Part model, mm, in its own coordinate system. A direction names the side the tool comes from. Give positions to 0.01 mm unless a question says otherwise; leave off trailing zeros. Order: outer loops, then holes, each group sorted by start corner. A loop starts at its lowest first (then second) coordinate and runs counter-clockwise, first axis right, second up. Notation, with made-up numbers: M 19,51 L 30,51 A25 cw 30,82 Z; hole C 54,85.5 d1. An arc over 180 degrees is marked long. Return JSON: item names as keys, results as strings.
from build123d import *

# Parameters (mm, degrees)
F0_R     = 50.9
F0_R_2   = 40.9
F1_DEPTH = 12.7
F2_R     = 5
F3_R     = 42.5
F4_DEPTH = 10
F5_R     = 42.5
F6_DEPTH = 10
F7_R     = 9.779
F8_DEPTH = 5.4


with BuildPart() as f1:
    # F0 (on Front) → F1 (new body, symmetric)
    with BuildSketch(Plane.XZ):
        Circle(F0_R)
        Circle(F0_R_2, mode=Mode.SUBTRACT)
        Circle(F0_R_2)
    extrude(amount=F1_DEPTH, both=True)

    # F2
    f2_edges = [f1.edges().sort_by_distance(p)[0] for p in [
        (-50.9, -12.7, 0),
        (-50.9, 12.7, 0),
    ]]
    fillet(f2_edges, radius=F2_R)

    # F3 (on face) → F4 (cut)
    with BuildSketch(Plane.XZ.offset(12.7)):
        Circle(F3_R)
    extrude(amount=-F4_DEPTH, mode=Mode.SUBTRACT)

    # F5 (on face) → F6 (cut)
    with BuildSketch(Plane(origin=(0, 12.7, 0), x_dir=(-1, 0, 0), z_dir=(0, 1, 0))):
        Circle(F5_R)
    extrude(amount=-F6_DEPTH, mode=Mode.SUBTRACT)

    # F7 (on face) → F8 (cut, through all)
    with BuildSketch(Plane.XZ.offset(2.7)):
        Circle(F7_R)
    extrude(amount=-F8_DEPTH, mode=Mode.SUBTRACT)


solid = f1.part
Q1. Band-saw the part on B-B (z = 0). Give the cut face in (x, y).
Established:
{"outline": "M -50.9,-7.7 A5 ccw -45.9,-12.7 L -42.5,-12.7 L -42.5,-2.7 L -9.78,-2.7 L -9.78,2.7 L -42.5,2.7 L -42.5,12.7 L -45.9,12.7 A5 ccw -50.9,7.7 Z; M 9.78,-2.7 L 42.5,-2.7 L 42.5,-12.7 L 45.9,-12.7 A5 ccw 50.9,-7.7 L 50.9,7.7 A5 ccw 45.9,12.7 L 42.5,12.7 L 42.5,2.7 L 9.78,2.7 Z"}
Q2. Band-saw the part on C-C (y = 5.5). Give the cut face in (x, z), then the cut area to 3 significant figures.
Established:
{"outline": "C 0,0 d101.8; hole C 0,0 d85", "area": "2,460 mm²"}
Q3. Two-plate mould, pull along Z, no slides. Class faces 1 (the flat face through (10, 2.7, 1)), 2 (the cylindrical face through (33.727, 7.77, -25.861)), 3 (the cylindrical face through (27.36, -0.11, 42.92)), 4 (the flat face through (13, -12.7, -41)): +Z half, -Z half, draft (parallel to the pull), parting line (faces both ways), or undercut.
Established:
{"face 1": "undercut", "face 2": "undercut", "face 3": "parting line", "face 4": "draft"}
Q4. Band-saw the part on A-A (x = 0). Give the cut face in (y, z).
Established:
{"outline": "M -12.7,-45.9 A5 ccw -7.7,-50.9 L 7.7,-50.9 A5 ccw 12.7,-45.9 L 12.7,-42.5 L 2.7,-42.5 L 2.7,-9.78 L -2.7,-9.78 L -2.7,-42.5 L -12.7,-42.5 Z; M -12.7,42.5 L -2.7,42.5 L -2.7,9.78 L 2.7,9.78 L 2.7,42.5 L 12.7,42.5 L 12.7,45.9 A5 ccw 7.7,50.9 L -7.7,50.9 A5 ccw -12.7,45.9 Z"}
Q5. Probe line 1 along Z through (x, y) = (0, 7.75); line 2 along Z through (x, y) = (0, 1); line 3 along Y through (x, z) = (13.5, 1). List the from-to ranges inside material, lowest first.
Established:
{"line 1": "z = -50.9 to -42.5, 42.5 to 50.9", "line 2": "z = -50.9 to -9.78, 9.78 to 50.9", "line 3": "y = -2.7 to 2.7"}
Q6. Band-saw the part on D-D (y = -9.5). Give the cut face in (x, z), then the cut area to 3 significant figures.
Established:
{"outline": "C 0,0 d101.13; hole C 0,0 d85", "area": "2,360 mm²"}
Q7. Pin check, flat tips, straight feed: pin 1 (8 mm diameter, centred on y = -10, z = 33, fed in from -X); pin 2 (8 mm diameter, centred on x = -35, y = 0, fed in from -Z); pin 3 (10 mm diameter, centred on y = 9.5, z = -18, fed in from -X); pin 4 (3 mm diameter, centred on y = 7.5, z = 1.5, fed in from -X). Stop position of each tip, or through.
Established:
{"pin 1": "stops at x = -41.56", "pin 2": "stops at z = -40.37", "pin 3": "stops at x = -49.14", "pin 4": "stops at x = -50.9"}
Q8. 3-axis set-ups, long thin cutter, end or side, ignore diameter. For faces 5 (the flat face through (-10, -2.7, 1)), 6 (the flat face through (13, 12.7, -41)): which of +Z, -Z, +X, -X, +Y, -Y reach the whole face in a straight line?
Established:
{"face 5": "-Y", "face 6": "+Z, -Z, +X, -X, +Y"}
